Source: CAD feature listing. Evaluate the final solid. Frame: model axes, mm. A direction names the side the tool comes from. Round coordinates to 2 decimals unless told otherwise and drop trailing zeros. Loops run counter-clockwise (first coordinate to the right, second up) from the corner with the lowest first, then second, coordinate; pieces in that order, holes last. Notation, with made-up numbers: (10.5, 42) - (14.5, 42) arc R27 ccw to (14.5, 76) - close; hole circle Ø3 at (41, 55). An arc over 180 degrees is marked (long way). One line per question, with ' | ' between items.
from build123d import *
from build123d.topology import SkipClean

# Parameters (mm, degrees)
CROQUIS1_R              = 2.5
CROQUIS1_R_2            = 2
SALIENTE_EXTRUIR1_DEPTH = 15
CROQUIS2_R              = 2.5
SALIENTE_EXTRUIR2_DEPTH = 1.2
CORTAR_EXTRUIR1_START   = -1.2
CORTAR_EXTRUIR1_DEPTH   = 1.2


with BuildPart() as part:
    # Croquis1 → Saliente-Extruir1 (new body)
    with BuildSketch(Plane.XY):
        Circle(CROQUIS1_R)
        Circle(CROQUIS1_R_2, mode=Mode.SUBTRACT)
    extrude(amount=SALIENTE_EXTRUIR1_DEPTH)

    # Croquis2 → Saliente-Extruir2 (add)
    with BuildSketch(Plane.XY.offset(15)):
        Circle(CROQUIS2_R)
    extrude(amount=SALIENTE_EXTRUIR2_DEPTH)

    # Croquis3 → Cortar-Extruir1 (cut)
    with SkipClean():  # the faces are left unmerged after this step: merging them gives an invalid solid
        with BuildSketch(Plane.XY.offset(16.2).offset(CORTAR_EXTRUIR1_START)):
            with BuildLine():
                Line((2, 0), (-2, 0))
                ThreePointArc((-2, 0), (0, 2), (2, 0))
            make_face()
        extrude(amount=CORTAR_EXTRUIR1_DEPTH, mode=Mode.SUBTRACT)


solid = part.part
1. Section query A-A, the plane x = -1.8. Return loops of the section in (y, z).
Worked out:
outline: (-1.73, 0) - (-0.87, 0) - (-0.87, 15) - (0, 15) - (0, 16.2) - (-1.73, 16.2) - close; (0.87, 0) - (1.73, 0) - (1.73, 16.2) - (0.87, 16.2) - close
2. Material intervals for probe 1 along Y at (x, z) = (0, 15.25); probe 2 along X at (y, z) = (-0.1, 5.75), sorted ascending.
Worked out:
probe 1: y = -2.5 to 0, 2 to 2.5 | probe 2: x = -2.5 to -2, 2 to 2.5
3. Contact query for flat-ended pins moving along their axis: P1, Ø1, axis at x = 0, y = -1, coming from the -Z side; P2, Ø1, axis at y = -1.5, z = 14.5, coming from the +X side; P3, Ø0.6, axis at x = -0.5, z = 15.5, coming from the +Y side. Output: stop coordinate, or through.
Worked out:
P1: stops at z = 15 | P2: stops at x = 2.29 | P3: stops at y = 2.49
4. Section query B-B, the plane y = 0.9. Return loops of the section in (x, z).
Worked out:
outline: (-2.33, 0) - (-1.79, 0) - (-1.79, 16.2) - (-2.33, 16.2) - close; (1.79, 0) - (2.33, 0) - (2.33, 16.2) - (1.79, 16.2) - close
5. Mould query, pull axis X, two halves, no side actions, for faces 1 (the cylindrical face through (-0.54, -2.44, 7.99)), 2 (the flat face through (-1, 2, 0)), 3 (the flat face through (0, -1, 15)). Classes: released by +X, released by -X, zero draft, split by the parting line, or undercut.
Worked out:
face 1: split by the parting line | face 2: zero draft | face 3: undercut
6. Section query C-C, the plane z = 6.5. Return loops of the section in (x, y), plus the area to 3 significant figures.
Worked out:
outline: circle Ø5 at (0, 0); hole circle Ø4 at (0, 0) | area: 7.07 mm2
7. Section query D-D, the plane y = -0.65. Return loops of the section in (x, z).
Worked out:
outline: (-2.41, 0) - (-1.89, 0) - (-1.89, 15) - (1.89, 15) - (1.89, 0) - (2.41, 0) - (2.41, 16.2) - (-2.41, 16.2) - close
8. Access query for faces 4 (the flat face through (0, 0, 16)), 5 (the flat face through (0, -1, 16.2)). Directions: +Z, -Z, +X, -X, +Y, -Y. A direction counts if a zero-diameter tool reaches every point of the face in a straight line with its end or side. Return the directions, or none.
Worked out:
face 4: +Z, -Z | face 5: +Z, +X, -X, +Y, -Y
